from build123d import *

# Parameters (mm, degrees)
F0_W     = 200
F0_H     = 100
F0_R     = 25
F1_DEPTH = 50
F2_W     = 100
F2_H     = 100
F2_R     = 25
F3_DEPTH = 25


# Not quite as in the source:
# - a feature names something its author has since deleted; it is built from what else it names


with BuildPart() as f1:
    # F0 (on Top) → F1 (new body)
    with BuildSketch(Plane.XY):
        with Locations((12.7213582092, 1.0950192809)):
            Rectangle(F0_W, F0_H)
        Circle(F0_R, mode=Mode.SUBTRACT)
    extrude(amount=F1_DEPTH)

    # F2 (on face) → F3 (cut)
    with BuildSketch(Plane.XY.offset(50)):
        with Locations((12.7213582092, 1.0950192809)):
            Rectangle(F2_W, F2_H)
        Circle(F2_R, mode=Mode.SUBTRACT)
    extrude(amount=-F3_DEPTH, mode=Mode.SUBTRACT)


solid = f1.part
Build history of the part. All positions in model axes, mm. A direction names the side the tool comes from. Round coordinates to 2 decimals unless told otherwise and drop trailing zeros. Write each loop counter-clockwise with the first axis right and the second up, starting at its lowest first coordinate (ties: lowest second). Pieces come first, ordered by that corner, then holes. Notation, with made-up numbers: (30, 46) - (41, 46) arc R24 cw to (41, 58) - close; hole circle Ø1 at (13, -27.75). An arc over 180 degrees is marked (long way). One line per question, with ' | ' between items.
1. Band-saw the part on B-B, the plane x = 0. Write the cut outline in (y, z), and give its area (3 significant figures).
Results are:
outline: (-48.9, 0) - (-25, 0) - (-25, 25) - (-48.9, 25) - close; (25, 0) - (51.1, 0) - (51.1, 25) - (25, 25) - close | area: 1,250 mm^2
2. Drill centre lines: line 1 along X through (y, z) = (23, 40); line 2 along Y through (x, z) = (0, 18); line 3 along Z through (x, y) = (-33, -7). Where is each one in solid material? Low to high. Write a range as from..to.
Results are:
line 1: -87.28..-37.28, 62.72..112.72 | line 2: -48.9..-25, 25..51.1 | line 3: 0..25
3. Drop flat-ended pins along their axis: pin 1 Ø10 at (x, y) = (60, 30.5) entering from +Z; pin 2 Ø2 at (x, y) = (-19.5, 21) entering from +Z. Give the stop position or say it passes through.
Results are:
pin 1: z = 50 | pin 2: z = 25
4. Band-saw the part on A-A, the plane z = 34.5. Write the cut outline in (x, y), and give its area (3 significant figures).
Results are:
outline: (-87.28, -48.9) - (-37.28, -48.9) - (-37.28, 51.1) - (-87.28, 51.1) - close; (62.72, -48.9) - (112.72, -48.9) - (112.72, 51.1) - (62.72, 51.1) - close | area: 10,000 mm^2
5. Mould opens along X. For faces 3 (the face through (62.721, 0, 38)), 4 (the face through (87, 2, 50)), 5 (the face through (-87.279, 0, 25)) say: released by +X, released by -X, zero draft, split by the parting line, or undercut.
Results are:
face 3: undercut | face 4: zero draft | face 5: released by -X
6. Tool access for faces 1 (the face through (-63, 2, 50)), 2 (the face through (23, 13, 25)): list every direction of +Z, -Z, +X, -X, +Y, -Y with a clear straight run to the whole face (end or side of a thin tool).
Results are:
face 1: +Z, +X, -X, +Y, -Y | face 2: +Z, +Y, -Y
7. Band-saw the part on D-D, the plane y = -39.5. Write the cut outline in (x, z), and give its area (3 significant figures).
Results are:
outline: (-87.28, 0) - (112.72, 0) - (112.72, 50) - (62.72, 50) - (62.72, 25) - (-37.28, 25) - (-37.28, 50) - (-87.28, 50) - close | area: 7,500 mm^2
8. Band-saw the part on C-C, the plane y = 0. Write the cut outline in (x, z), and give its area (3 significant figures).
Results are:
outline: (-87.28, 0) - (-25, 0) - (-25, 25) - (-37.28, 25) - (-37.28, 50) - (-87.28, 50) - close; (25, 0) - (112.72, 0) - (112.72, 50) - (62.72, 50) - (62.72, 25) - (25, 25) - close | area: 6,250 mm^2
